Geometry: final body of the model. Coordinates: model frame, mm. Round coordinates to 2 decimals unless told otherwise and drop trailing zeros. Loops run counter-clockwise (first coordinate to the right, second up) from the corner with the lowest first, then second, coordinate; pieces in that order, holes last. Notation, with made-up numbers: (9.25, 67.5) -> (65.25, 67.5) arc R15 ccw to (65.25, 81.5) -> close; hole circle Ø4 at (46.5, 63.25). An arc over 180 degrees is marked (long way). Answer in a Markdown table with one row per item.
```python
from build123d import *

# Parameters (mm, degrees)
MODEL_R                 = 4.984012051
MODEL_W                 = 19.932346667
MODEL_H                 = 3
SALIENTE_EXTRUIR1_DEPTH = 3


with BuildPart() as part:
    # Model → Saliente-Extruir1 (new body)
    with BuildSketch(Plane.XY):
        Polygon((86.791955129, -43.830425543), (2.925288462, -43.830425543), (2.925288462, 34.469098382), (2.925288462, 74.169574457), (86.791955129, 74.169574457), align=None)
        with Locations((37.750400228, 42.990457696)):
            Circle(MODEL_R, mode=Mode.SUBTRACT)
        with Locations((58.835741796, 64.469574457)):
            Rectangle(MODEL_W, MODEL_H, mode=Mode.SUBTRACT)
        with Locations((30.881501796, 64.469574457)):
            Rectangle(MODEL_W, MODEL_H, mode=Mode.SUBTRACT)
    extrude(amount=SALIENTE_EXTRUIR1_DEPTH)


solid = part.part
```
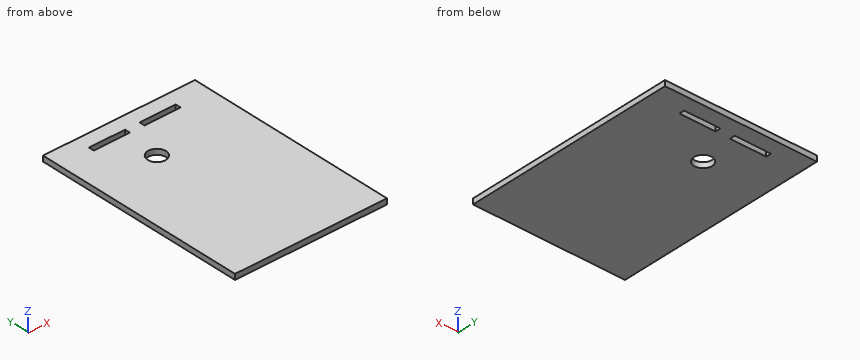
Item 1: Pin query (flat end, axial travel): pin 1 Ø4 at (x, y) = (53.5, 28.5) entering from -Z. Return the tip coordinate at first contact, or that it passes through.
Answer:
| item | result |
|---|---|
| pin 1 | stops at z = 0 |
Item 2: Cut plane C-C (z = 1.3). Output: boundary loops of the cut face in (x, y), then the cut area to 3 significant figures.
Answer:
| item | result |
|---|---|
| outline | (2.93, -43.83) -> (86.79, -43.83) -> (86.79, 74.17) -> (2.93, 74.17) -> close; hole (20.92, 62.97) -> (40.85, 62.97) -> (40.85, 65.97) -> (20.92, 65.97) -> close; hole circle Ø9.97 at (37.75, 42.99); hole (48.87, 62.97) -> (68.8, 62.97) -> (68.8, 65.97) -> (48.87, 65.97) -> close |
| area | 9,700 mm² |
Item 3: Line query: probe 1 along Y at (x, z) = (56, 1.55); probe 2 along Y at (x, z) = (37, 2.55); probe 3 along X at (y, z) = (42.5, 1). Output: solid intervals per line, ascending. Write a range as [from, to].
Answer:
| item | result |
|---|---|
| probe 1 | y = [-43.83, 62.97], [65.97, 74.17] |
| probe 2 | y = [-43.83, 38.06], [47.92, 62.97], [65.97, 74.17] |
| probe 3 | x = [2.93, 32.79], [42.71, 86.79] |
Item 4: Cut plane B-B (x = 38). Output: boundary loops of the cut face in (y, z).
Answer:
| item | result |
|---|---|
| outline | (-43.83, 0) -> (38.01, 0) -> (38.01, 3) -> (-43.83, 3) -> close; (47.97, 0) -> (62.97, 0) -> (62.97, 3) -> (47.97, 3) -> close; (65.97, 0) -> (74.17, 0) -> (74.17, 3) -> (65.97, 3) -> close |
Item 5: Cut plane A-A (x = 53). Output: boundary loops of the cut face in (y, z).
Answer:
| item | result |
|---|---|
| outline | (-43.83, 0) -> (62.97, 0) -> (62.97, 3) -> (-43.83, 3) -> close; (65.97, 0) -> (74.17, 0) -> (74.17, 3) -> (65.97, 3) -> close |
